Build history of the part. All positions in model axes, mm. Face numbers are marked on the shaded views. Coordinates: 2 decimals unless noted, no trailing zeros. Order: outer loops, then holes, each group sorted by start corner. A loop starts at its lowest first (then second) coordinate and runs counter-clockwise, first axis right, second up. Notation, with made-up numbers: M -14.5,19 L -2.5,19 A36 cw -2.5,57 Z; hole C -36.75,-30 d8. An arc over 180 degrees is marked long. Use a Markdown table: item, result. Add a question column.
from build123d import *

# Parameters (mm, degrees)
FILLET2_R          = 1
SKETCH2_R          = 11.696559432
CUT_EXTRUDE1_DEPTH = 206


with BuildPart() as part:
    # Sketch1 → Revolve1 (revolve)
    with BuildSketch(Plane.XY):
        Polygon((0, 0), (0, 200), (15, 200), (15, 0), (25, 0), (25, -5), (0, -5), align=None)
    revolve(axis=Axis((0, 0, 0), (0, 1, 0)))

    # Fillet2
    fillet2_edges = [part.edges().sort_by_distance(p)[0] for p in [
        (-25, 0, 0),
    ]]
    fillet(fillet2_edges, radius=FILLET2_R)

    # Sketch2 → Cut-Extrude1 (cut, through all)
    with BuildSketch(Plane(origin=(0, 200, 0), x_dir=(1, 0, 0), z_dir=(0, 1, 0))):
        Circle(SKETCH2_R)
    extrude(amount=-CUT_EXTRUDE1_DEPTH, mode=Mode.SUBTRACT)


solid = part.part
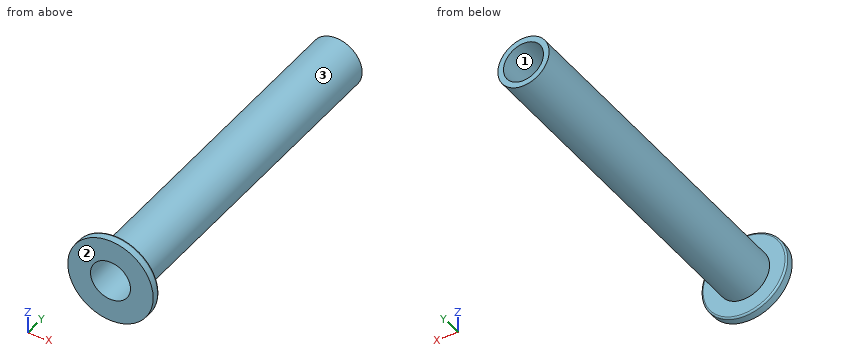
(1) Mould opens along Z. For the marked faces 1, 2 and 3 say: released by +Z, released by -Z, zero draft, split by the parting line, or undercut.
(2) Drop flat-ended pins along their axis: P1, Ø4, axis at y = 89, z = -9, coming from the +X side; P2, Ø3, axis at x = 18, y = 154, coming from the -Z side; P3, Ø24, axis at x = -9, z = 2, coming from the +Y side; P4, Ø3, axis at y = 104, z = -2, coming from the +X side. Give the stop position or say it passes through.
(3) Slice it at A-A on x = 0. Give the cut face in (y, z), and give its area (3 significant figures).
(4) Drill centre lines: line 1 along X through (y, z) = (144.5, 0); line 2 along Y through (x, z) = (-2.5, 21.5). Where is each one in solid material? Low to high. Write a range as from..to.
(5) Slice it at B-B on z = 0. Give the cut face in (x, y).
(6) Slice it at C-C on y = 69. Give the cut face in (x, z), and give its area (3 significant figures).
Solutions:
| question | item | result |
|---|---|---|
| 1 | face 1 | undercut |
| 1 | face 2 | zero draft |
| 1 | face 3 | split by the parting line |
| 2 | P1 | x = 13.27 |
| 2 | P2 | through |
| 2 | P3 | y = 200 |
| 2 | P4 | x = 14.99 |
| 3 | outline | M -5,-25 L -1,-25 A1 ccw 0,-24 L 0,-15 L 200,-15 L 200,-11.7 L -5,-11.7 Z; M -5,11.7 L 200,11.7 L 200,15 L 0,15 L 0,24 A1 ccw -1,25 L -5,25 Z |
| 3 | area | 1,450 mm² |
| 4 | line 1 | -15..-11.7, 11.7..15 |
| 4 | line 2 | -5..0 |
| 5 | outline | M -25,-5 L -11.7,-5 L -11.7,200 L -15,200 L -15,0 L -24,0 A1 ccw -25,-1 Z; M 11.7,-5 L 25,-5 L 25,-1 A1 ccw 24,0 L 15,0 L 15,200 L 11.7,200 Z |
| 6 | outline | C 0,0 d30; hole C 0,0 d23.39 |
| 6 | area | 277 mm² |
